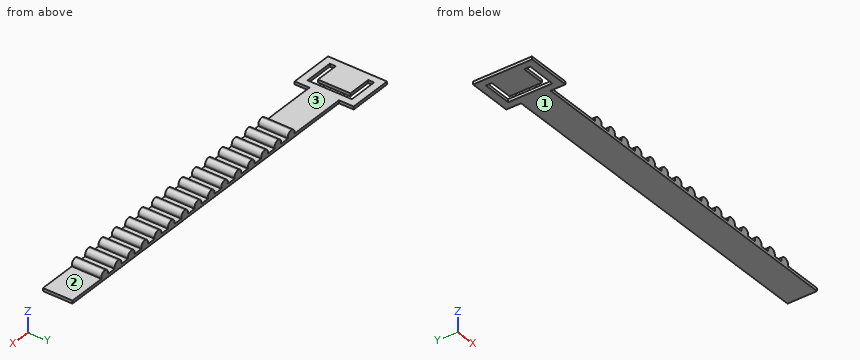
```python
from build123d import *

# Parameters (mm, degrees)
F0_W     = 120
F0_H     = 10
F1_DEPTH = 1
F2_W     = 3
F2_H     = 10
F3_DEPTH = 3
F4_R     = 1.5
F5_R     = 1.49999
F6_R     = 1.49999


# Not quite as in the source:
# - a fillet or chamfer is up to 0.001 mm smaller than in the source, because OpenCascade refuses the exact size


with BuildPart() as f1:
    # F0 (on Top) → F1 (new body)
    with BuildSketch(Plane.XY):
        Rectangle(F0_W, F0_H)
        Polygon((-60, -5), (-60, 5), (-60, 10), (-75, 10), (-75, -10), (-60, -10), align=None)
        Polygon((-72.5, 5.5), (-72.5, 7.5), (-62.5, 7.5), (-62.5, -7.5), (-72.5, -7.5), (-72.5, -5.5), (-64.5, -5.5), (-64.5, 5.5), align=None, mode=Mode.SUBTRACT)
    extrude(amount=F1_DEPTH)

    # F2 (on Top) → F3 (join)
    with BuildSketch(Plane.XY):
        with Locations((-38.5, 0)):
            Rectangle(F2_W, F2_H)
        with Locations((-32.5, 0)):
            Rectangle(F2_W, F2_H)
        with Locations((-26.5, 0)):
            Rectangle(F2_W, F2_H)
        with Locations((-20.5, 0)):
            Rectangle(F2_W, F2_H)
        with Locations((-14.5, 0)):
            Rectangle(F2_W, F2_H)
        with Locations((-8.5, 0)):
            Rectangle(F2_W, F2_H)
        with Locations((-2.5, 0)):
            Rectangle(F2_W, F2_H)
        with Locations((3.5, 0)):
            Rectangle(F2_W, F2_H)
        with Locations((9.5, 0)):
            Rectangle(F2_W, F2_H)
        with Locations((15.5, 0)):
            Rectangle(F2_W, F2_H)
        with Locations((21.5, 0)):
            Rectangle(F2_W, F2_H)
        with Locations((27.5, 0)):
            Rectangle(F2_W, F2_H)
        with Locations((33.5, 0)):
            Rectangle(F2_W, F2_H)
        with Locations((39.5, 0)):
            Rectangle(F2_W, F2_H)
        with Locations((45.5, 0)):
            Rectangle(F2_W, F2_H)
    extrude(amount=F3_DEPTH)

    # F4
    f4_edges = [f1.edges().sort_by_distance(p)[0] for p in [
        (-40, 0, 3),
    ]]
    fillet(f4_edges, radius=F4_R)

    # F5 (radius 1.5 in the source; OpenCascade refuses exactly that, so slightly less here)
    f5_edges = [f1.edges().sort_by_distance(p)[0] for p in [
        (-37, 0, 3),
    ]]
    fillet(f5_edges, radius=F5_R)

    # F6 (radius 1.5 in the source; OpenCascade refuses exactly that, so slightly less here)
    f6_edges = [f1.edges().sort_by_distance(p)[0] for p in [
        (-34, 0, 3),
        (-31, 0, 3),
        (-28, 0, 3),
        (-25, 0, 3),
        (-22, 0, 3),
        (-19, 0, 3),
        (-16, 0, 3),
        (-13, 0, 3),
        (-10, 0, 3),
        (-7, 0, 3),
        (-4, 0, 3),
        (-1, 0, 3),
        (2, 0, 3),
        (5, 0, 3),
        (8, 0, 3),
        (11, 0, 3),
        (14, 0, 3),
        (17, 0, 3),
        (20, 0, 3),
        (23, 0, 3),
        (26, 0, 3),
        (29, 0, 3),
        (32, 0, 3),
        (35, 0, 3),
        (38, 0, 3),
        (41, 0, 3),
        (44, 0, 3),
        (47, 0, 3),
    ]]
    fillet(f6_edges, radius=F6_R)


solid = f1.part
```
Geometry check sheet. Reference: the model listing, model coordinates, mm. Face numbers are marked on the shaded views. A direction names the side the tool comes from. Round coordinates to 2 decimals unless told otherwise and drop trailing zeros. Loops run counter-clockwise (first coordinate to the right, second up) from the corner with the lowest first, then second, coordinate; pieces in that order, holes last. Notation, with made-up numbers: M 40,37.5 L 53,37.5 A11 cw 53,58.5 Z; hole C -26,-29 d10. An arc over 180 degrees is marked long. Return JSON: item names as keys, results as strings. Group by question number.
(1) Go/stop test with flat-tipped pins: pin 1 (0.9 mm diameter, centred on x = 12, y = 1.5, fed in from +Z); pin 2 (1.1 mm diameter, centred on y = -6, z = 0.5, fed in from +X); pin 3 (6 mm diameter, centred on x = 33, y = 1, fed in from -Z); pin 4 (3.5 mm diameter, centred on x = -23, y = -2.5, fed in from +Z). Record where each tip stops, or that it passes through.
(2) Set-up check for the marked faces 1, 2 and 3: record each of +Z, -Z, +X, -X, +Y, -Y from which the full face is reachable in a straight line by a thin tool's end or side.
(3) Section check B-B, the plane z = 2.15. Give the number of separate pieces and of enclosed holes in the cut face, and give its area (3 significant figures).
(4) Scan lines: line 1 along X through (y, z) = (3.75, 0.75); line 2 along Z through (x, y) = (23.5, 3.5); line 3 along Y through (x, z) = (-8, 0.45). Record each from-to range of solid material in increasing order. Write a range as [from, to].
(5) Section check A-A, the plane x = -44.5. Enter the section's corners in (y, z).
Data:
{
 "1": {"pin 1": "z = 1", "pin 2": "x = -60", "pin 3": "z = 0", "pin 4": "z = 2.8"},
 "2": {"face 1": "-Z, +X, -X, +Y, -Y", "face 2": "+Z, +X, +Y, -Y", "face 3": "+Z, -X, +Y, -Y"},
 "3": {"separate pieces": "15", "enclosed holes": "0", "area": "406 mm²"},
 "4": {"line 1": "[-75, -64.5], [-62.5, 60]", "line 2": "[0, 1]", "line 3": "[-5, 5]"},
 "5": {"outline": "M -5,0 L 5,0 L 5,1 L -5,1 Z"}
}
